Geometry check sheet. Reference: the model listing, model coordinates, mm. Face numbers are marked on the shaded views. Coordinates: 2 decimals unless noted, no trailing zeros. Loops run counter-clockwise (first coordinate to the right, second up) from the corner with the lowest first, then second, coordinate; pieces in that order, holes last. Notation, with made-up numbers: (70, 22.25) - (128, 22.25) arc R17 ccw to (128, 42.25) - close; hole circle Ø7 at (10.5, 78.5). An arc over 180 degrees is marked (long way). Write item = value, one per line. Start each with the question number.
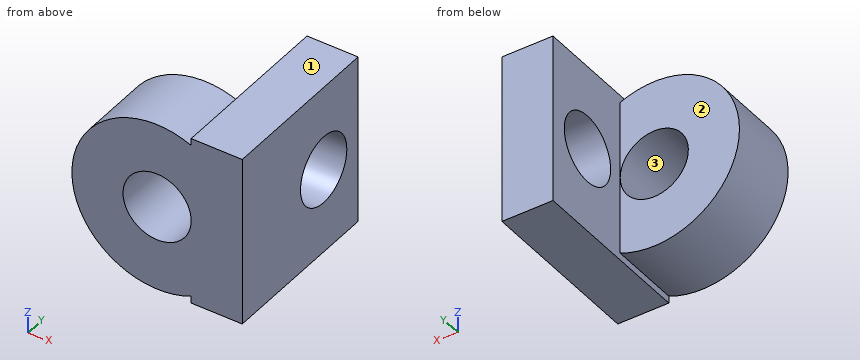
from build123d import *

# Parameters (mm, degrees)
SKETCH1_R           = 2.5
SKETCH1_R_2         = 1
BOSS_EXTRUDE2_DEPTH = 2.1
SKETCH2_W           = 5
SKETCH2_H           = 5
SKETCH2_R           = 1
BOSS_EXTRUDE3_DEPTH = 1.5


with BuildPart() as part:
    # Sketch1 → Boss-Extrude2 (new body)
    with BuildSketch(Plane(origin=(0, 0, 0), x_dir=(1, 0, 0), z_dir=(0, 1, 0))):
        with Locations(Location((0, 0, 0), (0, 0, 270))):
            Circle(SKETCH1_R)
        with Locations(Location((0, 0, 0), (0, 0, 270))):
            Circle(SKETCH1_R_2, mode=Mode.SUBTRACT)
    extrude(amount=BOSS_EXTRUDE2_DEPTH)

    # Sketch2 → Boss-Extrude3 (add)
    with BuildSketch(Plane(origin=(2.5, 0, 0), x_dir=(0, 0, -1), z_dir=(1, 0, 0))):
        with Locations((0, 2.5)):
            Rectangle(SKETCH2_W, SKETCH2_H)
        with Locations((0, 3.513067933)):
            Circle(SKETCH2_R, mode=Mode.SUBTRACT)
    extrude(amount=-BOSS_EXTRUDE3_DEPTH)


solid = part.part
(1) Sectioned sample at B-B on y = 4.1. Enter the section's corners in (x, z), plus the area to 3 significant figures.
(2) Scan lines: line 1 (X direction, y = 1.65, z = 0); line 2 (Y direction, x = 1.55, z = 0). Record each from-to range of solid material in increasing order.
(3) Sectioned sample at C-C on z = 0.3. Enter the section's corners in (x, y), plus the area to 3 significant figures.
(4) Draft check along Z on the marked faces 1, 2 and 3. Enter one of: pulls with the +Z half, pulls with the -Z half, needs draft (parallel to the pull), parting line crosses it, or undercut.
(5) Depth check by flat-ended pin: pin 1 (2 mm diameter, centred on x = -0.5, z = -1, fed in from +Y). Enter the tip coordinate at first touch or a pass-through.
(6) Sectioned sample at A-A on x = 0. Enter the section's corners in (y, z).
(7) Sectioned sample at D-D on y = 1.1. Enter the section's corners in (x, z), plus the area to 3 significant figures.
Working result:
q1.outline = (1, -2.5) - (2.5, -2.5) - (2.5, -0.81) - (1, -0.81) - close; (1, 0.81) - (2.5, 0.81) - (2.5, 2.5) - (1, 2.5) - close
q1.area = 5.07 mm2
q2.line_1 = -2.5 to -1, 1 to 2.5
q2.line_2 = 0 to 2.51, 4.51 to 5
q3.outline = (-2.48, 0) - (-0.95, 0) - (-0.95, 2.1) - (-2.48, 2.1) - close; (0.95, 0) - (2.5, 0) - (2.5, 2.56) - (1, 2.56) - (1, 2.1) - (0.95, 2.1) - close; (1, 4.47) - (2.5, 4.47) - (2.5, 5) - (1, 5) - close
q3.area = 7.94 mm2
q4.face_1 = pulls with the +Z half
q4.face_2 = needs draft
q4.face_3 = undercut
q5.pin_1 = 2.1
q6.outline = (0, -2.5) - (2.1, -2.5) - (2.1, -1) - (0, -1) - close; (0, 1) - (2.1, 1) - (2.1, 2.5) - (0, 2.5) - close
q7.outline = (1, -2.5) - (2.5, -2.5) - (2.5, 2.5) - (1, 2.5) - (1, 2.29) arc R2.5 ccw (long way) to (1, -2.29) - close; hole circle Ø2 at (0, 0)
q7.area = 19.0 mm2
